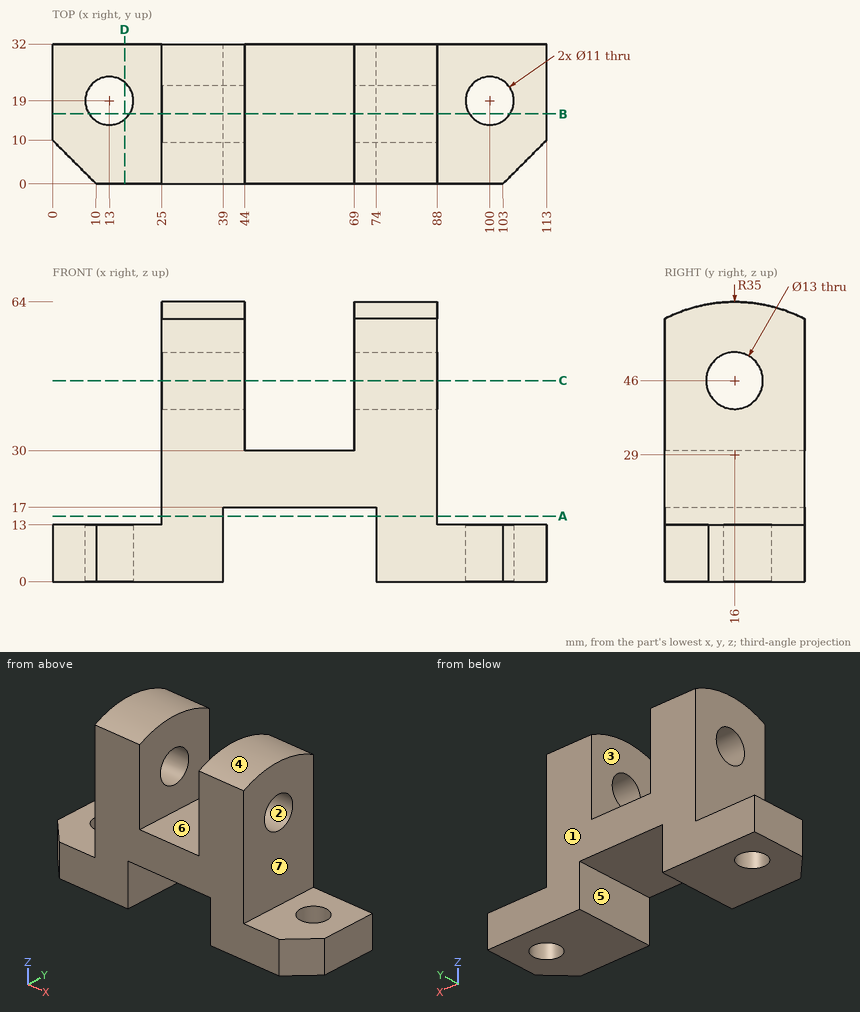
Answer from the drawing. Dimensions are ordinates in mm from the lowest x, y and z of the part. A direction names the side the tool comes from. Coordinates: 2 decimals unless noted, no trailing zeros. Order: outer loops, then holes, each group sorted by start corner. A loop starts at its lowest first (then second) coordinate and runs counter-clockwise, first axis right, second up. Notation, with made-up numbers: M 13.25,2.5 L 72.25,2.5 A23 ccw 72.25,14.5 Z; hole C 26.5,-0.5 d5. An arc over 180 degrees is marked long. Put each result on its own line as item: value. Start each with the question number.
Item 1: Section A-A, the plane z = 15 is taken. Determine the outline of the cut face in (x, y), plus the area to 3 significant figures.
Item 2: The mould has two halves that part along Y. Classify the marked faces 1, 2, 3 and 4: +Y half, -Y half, draft (parallel to the pull), parting line (faces both ways), or undercut.
Item 3: For the marked faces 5, 6 and 7, determine the directions among +Z, -Z, +X, -X, +Y, -Y from which every point of the face is accessible in a straight line to the end or side of a thin tool.
Item 4: Consider probe 1 along Y at (x, z) = (13, 9); probe 2 along X at (y, z) = (23, 47); probe 3 along X at (y, z) = (12.5, 11). Determine where each line is inside the solid, lowest interval first. Write a range as [from, to].
Item 5: Section D-D, the plane x = 16.5 is taken. Determine the outline of the cut face in (y, z).
Item 6: Section C-C, the plane z = 46 is taken. Determine the outline of the cut face in (x, y).
Item 7: Section B-B, the plane y = 16 is taken. Count the separate pieces of the cut face and the enclosed holes in it, plus the area to 3 significant figures.
Item 8: Given pin 1 Ø12 at (x, y) = (19.5, 8.5) entering from +Z; pin 2 Ø16 at (y, z) = (15.5, 53.5) entering from +X; pin 3 Ø7.5 at (x, y) = (16, 16.5) entering from +Z, each flat-ended and moving along its own axis, determine where each tip first touches the part or whether it passes through.
Computed:
1. outline: M 25,0 L 39,0 L 39,32 L 25,32 Z; M 74,0 L 88,0 L 88,32 L 74,32 Z
1. area: 896 mm2
2. face 1: +Y half
2. face 2: undercut
2. face 3: draft
2. face 4: parting line
3. face 5: -Z, +Y, -Y
3. face 6: +Z, +Y, -Y
3. face 7: +Z, +X, +Y, -Y
4. probe 1: y = [0, 13.5], [24.5, 32]
4. probe 2: x = [25, 44], [69, 88]
4. probe 3: x = [0, 39], [74, 113]
5. outline: M 0,0 L 14.76,0 L 14.76,13 L 0,13 Z; M 23.24,0 L 32,0 L 32,13 L 23.24,13 Z
6. outline: M 25,0 L 44,0 L 44,9.5 L 25,9.5 Z; M 25,22.5 L 44,22.5 L 44,32 L 25,32 Z; M 69,0 L 88,0 L 88,9.5 L 69,9.5 Z; M 69,22.5 L 88,22.5 L 88,32 L 69,32 Z
7. separate pieces: 5
7. enclosed holes: 0
7. area: 2,500 mm2
8. pin 1: stops at z = 63.63
8. pin 2: stops at x = 88
8. pin 3: stops at z = 13
